Could you check a few things on this model? Use its own coordinates, in mm. A direction names the side the tool comes from. Coordinates: 2 decimals unless noted, no trailing zeros. Order: outer loops, then holes, each group sorted by start corner. A loop starts at its lowest first (then second) coordinate and runs counter-clockwise, first axis right, second up. Notation, with made-up numbers: (-6.75, 84.25) - (24.25, 84.25) arc R23 cw to (24.25, 98.25) - close; hole circle Ø8 at (14, -34.5). An arc over 180 degrees is marked (long way). One line per item, written item: value. Start each with the question number.
from build123d import *

# Parameters (mm, degrees)
SKETCH1_R           = 1.75
BOSS_EXTRUDE1_DEPTH = 1.5


with BuildPart() as part:
    # Sketch1 → Boss-Extrude1 (new body)
    with BuildSketch(Plane.XY):
        with BuildLine():
            Line((4, -6), (-4, -6))
            Line((-4, -6), (-4, 8))
            Line((-4, 8), (11, 8))
            Line((11, 8), (11, 0))
            Line((11, 0), (6, 0))
            ThreePointArc((6, 0), (4.585786438, -0.585786438), (4, -2))
            Line((4, -2), (4, -6))
        make_face()
        Circle(SKETCH1_R, mode=Mode.SUBTRACT)
    extrude(amount=BOSS_EXTRUDE1_DEPTH)


solid = part.part
Q1. If I drill on L1, parallel to Y at x = 0, z = 0.75; L2, parallel to Y at x = 7.5, z = 0.6; L3, parallel to X at y = -1.25, z = 0.1, over which ranges is the centre line in solid material (lowest first)?
Q2. Which directions (+Z, -Z, +X, -X, +Y, -Y) give clear straight access to the entire face, cutting with the end or side of a thin tool? Please do faces 1 (the flat face through (9, 0, 1)), 2 (the flat face through (2, 3, 0)).
Q3. I want a section at A-A on x = 0. Please give me the cut outline in (y, z).
Q4. I'm going to push a flat-ended pin straight in: pin 1 (0.8 mm diameter, centred on y = -3.5, z = 0.5, fed in from +X). Where does the tip first touch, or does it pass through?
Q5. I want a section at D-D on x = 8.5. Please give me the cut outline in (y, z), then the cut area to 3 significant figures.
Q6. I want a section at C-C on y = -4.75. Please give me the cut outline in (x, z), then the cut area to 3 significant figures.
Q7. I want a section at B-B on z = 0.7. Please give me the cut outline in (x, y).
Values follow:
1. L1: y = -6 to -1.75, 1.75 to 8
1. L2: y = 0 to 8
1. L3: x = -4 to -1.22, 1.22 to 4.15
2. face 1: +Z, -Z, +X, -Y
2. face 2: -Z, +X, -X, +Y, -Y
3. outline: (-6, 0) - (-1.75, 0) - (-1.75, 1.5) - (-6, 1.5) - close; (1.75, 0) - (8, 0) - (8, 1.5) - (1.75, 1.5) - close
4. pin 1: stops at x = 4
5. outline: (0, 0) - (8, 0) - (8, 1.5) - (0, 1.5) - close
5. area: 12.0 mm^2
6. outline: (-4, 0) - (4, 0) - (4, 1.5) - (-4, 1.5) - close
6. area: 12.0 mm^2
7. outline: (-4, -6) - (4, -6) - (4, -2) arc R2 cw to (6, 0) - (11, 0) - (11, 8) - (-4, 8) - close; hole circle Ø3.5 at (0, 0)
